Check sheet for the modelled part. Datum: model origin and axes. Units: mm. Round coordinates to 2 decimals unless told otherwise and drop trailing zeros. Write each loop counter-clockwise with the first axis right and the second up, starting at its lowest first coordinate (ties: lowest second). Pieces come first, ordered by that corner, then holes. Notation, with made-up numbers: (-26, 19.25) -> (33, 19.25) arc R17 ccw to (33, 51.25) -> close; hole circle Ø4 at (54.5, -23). An arc over 180 degrees is marked (long way). One line per item, written item: value.
from build123d import *

# Parameters (mm, degrees)
ESQUISSE1_R        = 2.75
BOSS_EXTRU_1_DEPTH = 7
CHANFREIN1_SIZE    = 3


with BuildPart() as part:
    # Esquisse1 → Boss.-Extru.1 (new body)
    with BuildSketch(Plane.XY):
        with BuildLine():
            Line((0, -7.5), (25.5, -7.5))
            ThreePointArc((25.5, -7.5), (33, 0), (25.5, 7.5))
            Line((25.5, 7.5), (0, 7.5))
            ThreePointArc((0, 7.5), (-7.5, 0), (0, -7.5))
        make_face()
        Circle(ESQUISSE1_R, mode=Mode.SUBTRACT)
        with Locations((25.5, 0)):
            Circle(ESQUISSE1_R, mode=Mode.SUBTRACT)
    extrude(amount=BOSS_EXTRU_1_DEPTH)

    # Chanfrein1
    chanfrein1_edges = [part.edges().sort_by_distance(p)[0] for p in [
        (-2.75, 0, 7),
        (22.75, 0, 7),
    ]]
    chamfer(chanfrein1_edges, length=CHANFREIN1_SIZE)


solid = part.part
Item 1: Mould release check, pull along Y, two halves, no side actions. Record for faces 1 (the conical face through (-2.935, 0.129, 4.188)), 2 (the flat face through (13, 7.5, 3)), 3 (the flat face through (13, -7.5, 3)), 4 (the cylindrical face through (33, 0, 3)): pulls with the +Y half, pulls with the -Y half, needs draft (parallel to the pull), parting line crosses it, or undercut.
Answer:
face 1: undercut
face 2: pulls with the +Y half
face 3: pulls with the -Y half
face 4: parting line crosses it
Item 2: Depth check by flat-ended pin: P1, Ø2, axis at y = 3, z = 4.5, coming from the -X side; P2, Ø1, axis at y = -6, z = 3, coming from the +X side. Enter the tip coordinate at first touch or a pass-through.
Answer:
P1: stops at x = -7.23
P2: stops at x = 30.6
Item 3: Sectioned sample at A-A on y = 0. Enter the section's corners in (x, z).
Answer:
outline: (-7.5, 0) -> (-2.75, 0) -> (-2.75, 4) -> (-5.75, 7) -> (-7.5, 7) -> close; (2.75, 0) -> (22.75, 0) -> (22.75, 4) -> (19.75, 7) -> (5.75, 7) -> (2.75, 4) -> close; (28.25, 0) -> (33, 0) -> (33, 7) -> (31.25, 7) -> (28.25, 4) -> close
Item 4: Sectioned sample at B-B on z = 3. Enter the section's corners in (x, y), and give its area (3 significant figures).
Answer:
outline: (0, -7.5) -> (25.5, -7.5) arc R7.5 ccw to (25.5, 7.5) -> (0, 7.5) arc R7.5 ccw to start; hole circle Ø5.5 at (0, 0); hole circle Ø5.5 at (25.5, 0)
area: 512 mm^2
Item 5: Thickness scan on line 1 (Y direction, x = 25.5, z = 2.2); line 2 (X direction, y = 1.5, z = 3.75); line 3 (Z direction, x = 21, y = 0). Record the ranges inside material, lowest first.
Answer:
line 1: y = -7.5 to -2.75, 2.75 to 7.5
line 2: x = -7.35 to -2.3, 2.3 to 23.2, 27.8 to 32.85
line 3: z = 0 to 5.75
